```python
from build123d import *

# Parameters (mm, degrees)
SKETCH1_W               = 6.5
SKETCH1_H               = 6.5
BOSS_EXTRUDE1_DEPTH     = 35
CUT_EXTRUDE1_DEPTH      = 37.187014245
CUT_EXTRUDE1_DEPTH_BACK = 37.187014245
SKETCH2_W               = 2.5
SKETCH2_H               = 2.5


with BuildPart() as part:
    # Sketch1 → Boss-Extrude1 (new body)
    with BuildSketch(Plane(origin=(0, 0, 0), x_dir=(1, 0, 0), z_dir=(0, 1, 0))):
        with Locations((3.25, -3.25)):
            Rectangle(SKETCH1_W, SKETCH1_H)
    extrude(amount=BOSS_EXTRUDE1_DEPTH)

    # Sketch2 → Cut-Extrude1 (cut, two sides: drawn at the far end of the back side and taken through both)
    with BuildSketch(Plane(origin=(0, 35, 0), x_dir=(1, 0, 0), z_dir=(0, 1, 0)).offset(-CUT_EXTRUDE1_DEPTH_BACK)):
        with Locations((3.25, -5.25)):
            Rectangle(SKETCH2_W, SKETCH2_H)
    extrude(amount=CUT_EXTRUDE1_DEPTH + CUT_EXTRUDE1_DEPTH_BACK, mode=Mode.SUBTRACT)


solid = part.part
```
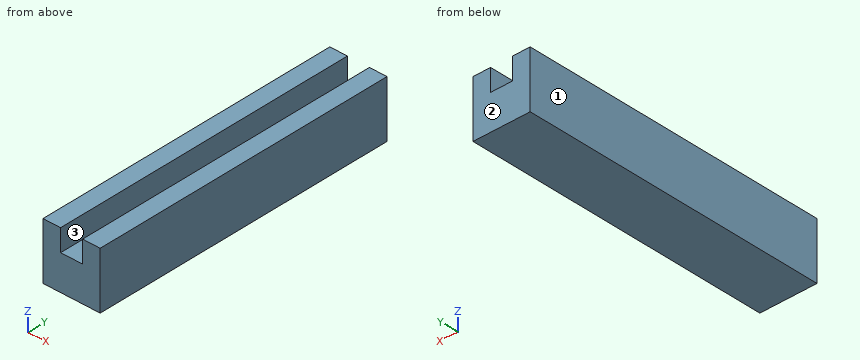
Model file for the job. Use its own axes, mm. Face numbers are marked on the shaded views. Coordinates: 2 decimals unless noted, no trailing zeros. Loops run counter-clockwise (first coordinate to the right, second up) from the corner with the lowest first, then second, coordinate; pieces in that order, holes last. Notation, with made-up numbers: (-1, -25) - (4, -25) arc R32 ccw to (4, 6) - close; hole circle Ø9 at (-9, 38.25). An arc over 180 degrees is marked (long way). Answer as a JSON object with one key per item and string values. Group by question number.
(1) Two-plate mould, pull along X, no slides. Class the marked faces 1, 2 and 3: released by +X, released by -X, zero draft, split by the parting line, or undercut.
(2) Cut at C-C (x = 3.5). Give the cut face in (y, z).
(3) Flat gauge pin, fed straight in: pin 1 (0.8 mm diameter, centred on x = 3.5, y = 9.5, fed in from +Z). Where does the tip first touch, or does it go through?
(4) Probe line 1 along X through (y, z) = (11, 4.5); line 2 along Z through (x, y) = (3, 2). List the from-to ranges inside material, lowest first.
(5) Cut at A-A (z = 4.5). Give the cut face in (x, y), then the cut area to 3 significant figures.
(6) Cut at B-B (y = 21). Give the cut face in (x, z).
Geometry says:
{
 "1": {"face 1": "released by -X", "face 2": "zero draft", "face 3": "undercut"},
 "2": {"outline": "(0, 0) - (35, 0) - (35, 4) - (0, 4) - close"},
 "3": {"pin 1": "stops at z = 4"},
 "4": {"line 1": "x = 0 to 2, 4.5 to 6.5", "line 2": "z = 0 to 4"},
 "5": {"outline": "(0, 0) - (2, 0) - (2, 35) - (0, 35) - close; (4.5, 0) - (6.5, 0) - (6.5, 35) - (4.5, 35) - close", "area": "140 mm^2"},
 "6": {"outline": "(0, 0) - (6.5, 0) - (6.5, 6.5) - (4.5, 6.5) - (4.5, 4) - (2, 4) - (2, 6.5) - (0, 6.5) - close"}
}
